Verification items for this drawing (mm, ordinates from the low corner). A direction names the side the tool comes from. Coordinates: 2 decimals unless noted, no trailing zeros. Order: outer loops, then holes, each group sorted by start corner. A loop starts at its lowest first (then second) coordinate and runs counter-clockwise, first axis right, second up. Notation, with made-up numbers: (38.25, -26) -> (82.25, -26) arc R20 ccw to (82.25, -21) -> close; hole circle Ø9 at (54.5, -17). An arc over 180 degrees is marked (long way). Write each question's results on one line, items separated by ' | '. Start each with the question number.
(1) Set-up check for the marked faces 1 and 2: record each of +Z, -Z, +X, -X, +Y, -Y from which the full face is reachable in a straight line by a thin tool's end or side.
(2) Thickness scan on probe 1 along Y at (x, z) = (38.1, 6.25); probe 2 along X at (y, z) = (38.1, 8.75) (3 decimals). Record the ranges inside material, lowest first. Write a range as [from, to].
(3) Cross-section at A-A on y = 38.1. Enter the section's corners in (x, z) (3 decimals), and give its area (3 significant figures).
(4) Go/stop test with flat-tipped pins: pin 1 (1.5 mm diameter, centred on x = 61, z = 6, fed in from -Y); pin 2 (4 mm diameter, centred on y = 38, z = 13, fed in from +X) (3 decimals); pin 3 (2 mm diameter, centred on x = 31.5, z = 3.5, fed in from +Y); pin 4 (7.5 mm diameter, centred on x = 38.1, y = 38.1, fed in from -Z). Record where each tip stops, or that it passes through.
(5) Draft check along X on the marked faces 3, 4 and 5. Enter one of: +X half, -X half, draft (parallel to the pull), parting line (faces both ways), or undercut.
(6) Cross-section at C-C on z = 14.5. Enter the section's corners in (x, y) (3 decimals), and give its area (3 significant figures).
(7) Cross-section at D-D on x = 59.5. Enter the section's corners in (y, z).
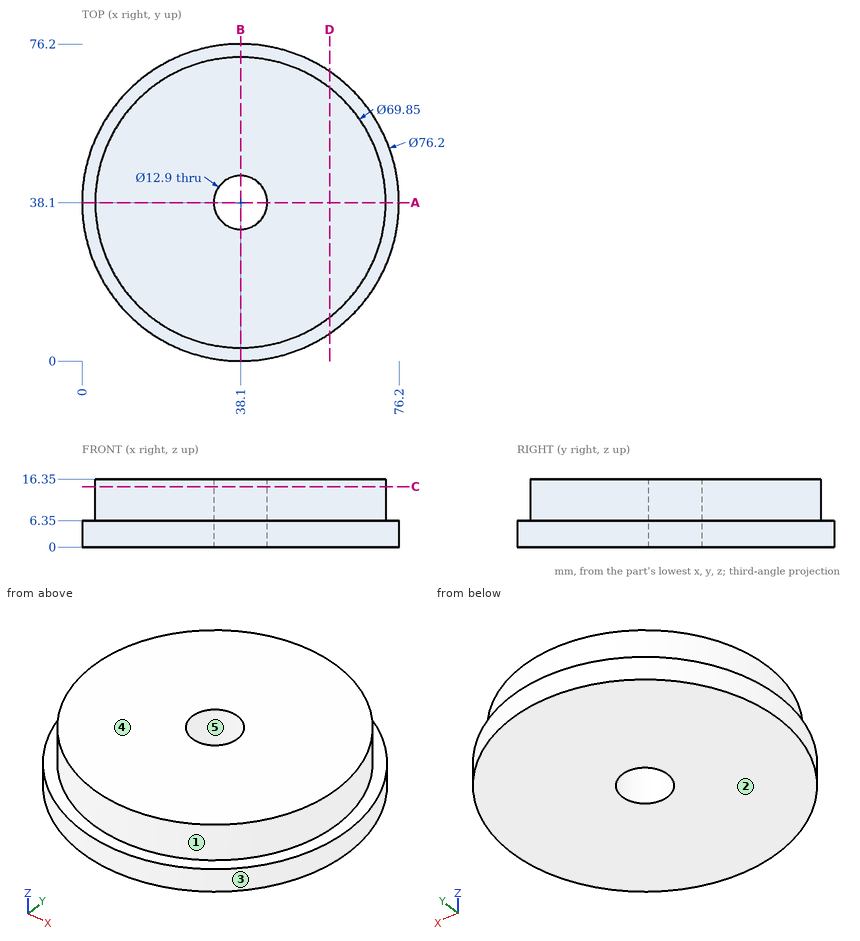
Results are:
1) face 1: +Z | face 2: -Z, +X, -X, +Y, -Y
2) probe 1: y = [0, 31.65], [44.55, 76.2] | probe 2: x = [3.175, 31.65], [44.55, 73.025]
3) outline: (0, 0) -> (31.65, 0) -> (31.65, 16.35) -> (3.175, 16.35) -> (3.175, 6.35) -> (0, 6.35) -> close; (44.55, 0) -> (76.2, 0) -> (76.2, 6.35) -> (73.025, 6.35) -> (73.025, 16.35) -> (44.55, 16.35) -> close | area: 971 mm2
4) pin 1: stops at y = 7.1 | pin 2: stops at x = 73.025 | pin 3: stops at y = 75.79 | pin 4: passes through
5) face 3: parting line | face 4: draft | face 5: undercut
6) outline: circle Ø69.85 at (38.1, 38.1); hole circle Ø12.9 at (38.1, 38.1) | area: 3,700 mm2
7) outline: (6.58, 0) -> (69.62, 0) -> (69.62, 6.35) -> (65.7, 6.35) -> (65.7, 16.35) -> (10.5, 16.35) -> (10.5, 6.35) -> (6.58, 6.35) -> close
